Build history of the part. All positions in model axes, mm. Give positions to 0.01 mm unless a question says otherwise; leave off trailing zeros. Write each loop counter-clockwise with the first axis right and the second up, starting at its lowest first coordinate (ties: lowest second). Pieces come first, ordered by that corner, then holes. Notation, with made-up numbers: M 81.25,83.5 L 108.25,83.5 A6 ccw 108.25,93.5 Z; hole C 54,-34.75 d2. An arc over 180 degrees is marked long. One line per item, written item: value. Start each with the question number.
from build123d import *

# Parameters (mm, degrees)
BOSS_EXTRUDE1_DEPTH                                  = 6
SKIZZE1_W                                            = 3
SKIZZE1_H                                            = 6
SCHNITT_LINEAR_AUSTRAGEN1_DEPTH                      = 722.828234416
FORMSENKUNG_FUR_M5_LINSENSENKSCHRAUBE_MI_D           = 5.5
FORMSENKUNG_FUR_M5_LINSENSENKSCHRAUBE_MI_CSINK_D     = 10.4
FORMSENKUNG_FUR_M5_LINSENSENKSCHRAUBE_MI_CSINK_ANGLE = 90
CHAMFER1_SIZE                                        = 1
CSK_FOR_M5_COUNTERSUNK_RAISED_HEAD_SCREW_D           = 5.5
CSK_FOR_M5_COUNTERSUNK_RAISED_HEAD_SCREW_CSINK_D     = 10.4
CSK_FOR_M5_COUNTERSUNK_RAISED_HEAD_SCREW_CSINK_ANGLE = 90
LPATTERN1_COUNT                                      = 7
LPATTERN1_PITCH                                      = 100
SPIEGELN1_COPY_1_D                                   = 5.5
SPIEGELN1_COPY_1_CSINK_D                             = 10.4
SPIEGELN1_COPY_1_CSINK_ANGLE                         = 90
SPIEGELN1_COPY_2_D                                   = 5.5
SPIEGELN1_COPY_2_CSINK_D                             = 10.4
SPIEGELN1_COPY_2_CSINK_ANGLE                         = 90
SPIEGELN1_COPY_3_D                                   = 5.5
SPIEGELN1_COPY_3_CSINK_D                             = 10.4
SPIEGELN1_COPY_3_CSINK_ANGLE                         = 90
SPIEGELN1_COPY_4_D                                   = 5.5
SPIEGELN1_COPY_4_CSINK_D                             = 10.4
SPIEGELN1_COPY_4_CSINK_ANGLE                         = 90
SPIEGELN1_COPY_5_D                                   = 5.5
SPIEGELN1_COPY_5_CSINK_D                             = 10.4
SPIEGELN1_COPY_5_CSINK_ANGLE                         = 90
SPIEGELN1_COPY_6_D                                   = 5.5
SPIEGELN1_COPY_6_CSINK_D                             = 10.4
SPIEGELN1_COPY_6_CSINK_ANGLE                         = 90


with BuildPart() as part:
    # Sketch1 → Boss-Extrude1 (new body)
    with BuildSketch(Plane(origin=(0, 0, 0), x_dir=(0, 0, -1), z_dir=(1, 0, 0))):
        with BuildLine():
            Line((-355, 130), (355, 130))
            Line((355, 130), (355, 33))
            Line((355, 33), (205, 33))
            ThreePointArc((205, 33), (190.354181484, 29.571946165), (178.751190503, 20))
            Line((178.751190503, 20), (138.751190503, 20))
            ThreePointArc((138.751190503, 20), (118.751190503, 0), (138.751190503, -20))
            Line((138.751190503, -20), (178.751190503, -20))
            ThreePointArc((178.751190503, -20), (190.354181484, -29.571946165), (205, -33))
            Line((205, -33), (355, -33))
            Line((355, -33), (355, -130))
            Line((355, -130), (-355, -130))
            Line((-355, -130), (-355, 130))
        make_face()
    extrude(amount=BOSS_EXTRUDE1_DEPTH)

    # Skizze1 → Schnitt-Linear austragen1 (cut, through all)
    with BuildSketch(Plane.XY.offset(355)):
        with Locations((4.5, -127)):
            Rectangle(SKIZZE1_W, SKIZZE1_H)
        with Locations((4.5, 127)):
            Rectangle(SKIZZE1_W, SKIZZE1_H)
    extrude(amount=-SCHNITT_LINEAR_AUSTRAGEN1_DEPTH, mode=Mode.SUBTRACT)

    # Formsenkung fur M5 Linsensenkschraube mit Schlitz1 (through all)
    with Locations(Plane.ZY):
        with Locations((349, -110), (349, -45)):
            formsenkung_fur_m5_linsensenkschraube_mi = CounterSinkHole(FORMSENKUNG_FUR_M5_LINSENSENKSCHRAUBE_MI_D / 2, FORMSENKUNG_FUR_M5_LINSENSENKSCHRAUBE_MI_CSINK_D / 2, counter_sink_angle=FORMSENKUNG_FUR_M5_LINSENSENKSCHRAUBE_MI_CSINK_ANGLE)

    # Chamfer1
    chamfer1_edges = [part.edges().sort_by_distance(p)[0] for p in [
        (6, 0, 355),
    ]]
    chamfer(chamfer1_edges, length=CHAMFER1_SIZE)

    # CSK for M5 Countersunk Raised Head Screw1 (through all)
    with Locations(Plane.ZY):
        with Locations((315, -109)):
            csk_for_m5_countersunk_raised_head_screw = CounterSinkHole(CSK_FOR_M5_COUNTERSUNK_RAISED_HEAD_SCREW_D / 2, CSK_FOR_M5_COUNTERSUNK_RAISED_HEAD_SCREW_CSINK_D / 2, counter_sink_angle=CSK_FOR_M5_COUNTERSUNK_RAISED_HEAD_SCREW_CSINK_ANGLE)

    # LPattern1: CSK for M5 Countersunk Raised Head Screw1 ×7
    with Locations(*[(0, 0, -i * LPATTERN1_PITCH) for i in range(1, LPATTERN1_COUNT)]):
        add(csk_for_m5_countersunk_raised_head_screw, mode=Mode.SUBTRACT)

    # Spiegeln1: Formsenkung fur M5 Linsensenkschraube mit Schlitz1, CSK for M5 Countersunk Raised Head Screw1 across plane
    add(formsenkung_fur_m5_linsensenkschraube_mi.mirror(Plane.ZX), mode=Mode.SUBTRACT)
    add(csk_for_m5_countersunk_raised_head_screw.mirror(Plane.ZX), mode=Mode.SUBTRACT)

    # Spiegeln1 copy 1 (through all)
    with Locations(Plane(origin=(0, 0, -100), x_dir=(0, 0, 1), z_dir=(-1, 0, 0))):
        with Locations((315, 109)):
            CounterSinkHole(SPIEGELN1_COPY_1_D / 2, SPIEGELN1_COPY_1_CSINK_D / 2, counter_sink_angle=SPIEGELN1_COPY_1_CSINK_ANGLE)

    # Spiegeln1 copy 2 (through all)
    with Locations(Plane(origin=(0, 0, -200), x_dir=(0, 0, 1), z_dir=(-1, 0, 0))):
        with Locations((315, 109)):
            CounterSinkHole(SPIEGELN1_COPY_2_D / 2, SPIEGELN1_COPY_2_CSINK_D / 2, counter_sink_angle=SPIEGELN1_COPY_2_CSINK_ANGLE)

    # Spiegeln1 copy 3 (through all)
    with Locations(Plane(origin=(0, 0, -300), x_dir=(0, 0, 1), z_dir=(-1, 0, 0))):
        with Locations((315, 109)):
            CounterSinkHole(SPIEGELN1_COPY_3_D / 2, SPIEGELN1_COPY_3_CSINK_D / 2, counter_sink_angle=SPIEGELN1_COPY_3_CSINK_ANGLE)

    # Spiegeln1 copy 4 (through all)
    with Locations(Plane(origin=(0, 0, -400), x_dir=(0, 0, 1), z_dir=(-1, 0, 0))):
        with Locations((315, 109)):
            CounterSinkHole(SPIEGELN1_COPY_4_D / 2, SPIEGELN1_COPY_4_CSINK_D / 2, counter_sink_angle=SPIEGELN1_COPY_4_CSINK_ANGLE)

    # Spiegeln1 copy 5 (through all)
    with Locations(Plane(origin=(0, 0, -500), x_dir=(0, 0, 1), z_dir=(-1, 0, 0))):
        with Locations((315, 109)):
            CounterSinkHole(SPIEGELN1_COPY_5_D / 2, SPIEGELN1_COPY_5_CSINK_D / 2, counter_sink_angle=SPIEGELN1_COPY_5_CSINK_ANGLE)

    # Spiegeln1 copy 6 (through all)
    with Locations(Plane(origin=(0, 0, -600), x_dir=(0, 0, 1), z_dir=(-1, 0, 0))):
        with Locations((315, 109)):
            CounterSinkHole(SPIEGELN1_COPY_6_D / 2, SPIEGELN1_COPY_6_CSINK_D / 2, counter_sink_angle=SPIEGELN1_COPY_6_CSINK_ANGLE)


solid = part.part
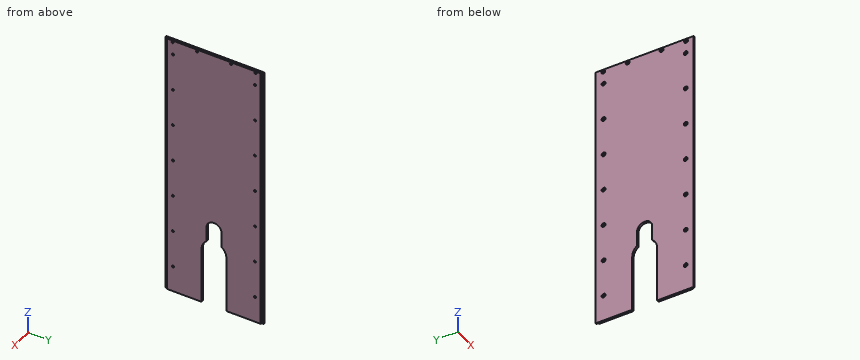
1) Band-saw the part on B-B (z = -69). List the corners of the cut face in (x, y), then the cut area to 3 significant figures.
2) Probe line 1 along Y through (x, z) = (3.2, 349); line 2 along Y through (x, z) = (4.8, 215); line 3 along Y through (x, z) = (3.8, -285). List the from-to ranges inside material, lowest first. Write a range as from..to.
3) Drop flat-ended pins along their axis: P1, Ø5, axis at y = -45, z = 349, coming from the -X side; P2, Ø5, axis at y = -128, z = -87, coming from the +X side; P3, Ø0.9, axis at x = 4.5, z = -102, coming from the -Y side; P4, Ø9, axis at y = 109, z = 315, coming from the -X side. Give the stop position or say it passes through.
4) Band-saw the part on A-A (x = 4). Count the separate pieces of the cut face and the enclosed holes in it, then the cut area to 3 significant figures.
Model answer:
1. outline: M 0,-130 L 3,-130 L 3,-124 L 6,-124 L 6,124 L 3,124 L 3,130 L 0,130 Z
1. area: 1,520 mm²
2. line 1: y = -124..-112.75, -107.25..-47.75, -42.25..42.25, 47.75..107.25, 112.75..124
2. line 2: y = -124..-111.75, -106.25..106.25, 111.75..124
2. line 3: y = -124..-111.75, -106.25..-33, 33..106.25, 111.75..124
3. P1: passes through
3. P2: stops at x = 3
3. P3: stops at y = -124
3. P4: stops at x = 0.7
4. separate pieces: 1
4. enclosed holes: 18
4. area: 162,000 mm²
